from build123d import *

# Parameters (mm, degrees)
IZIM1_R                     = 1.5
IZIM1_R_2                   = 1.5621
IZIM1_R_3                   = 2.5
Y_KSEKLIK_EKSTR_ZYON1_DEPTH = 3


with BuildPart() as part:
    # Çizim1 → Yükseklik-Ekstrüzyon1 (new body)
    with BuildSketch(Plane(origin=(0, 0, 0), x_dir=(1, 0, 0), z_dir=(0, 1, 0))):
        with BuildLine():
            Line((-78.950997289, 12.5), (-73.950997289, 12.5))
            ThreePointArc((-73.950997289, 12.5), (-53.033008589, 53.033008589), (-12.5, 73.950997289))
            Line((-12.5, 73.950997289), (-12.5, 78.950997289))
            ThreePointArc((-12.5, 78.950997289), (0, 91.450997289), (12.5, 78.950997289))
            Line((12.5, 78.950997289), (12.5, 73.950997289))
            ThreePointArc((12.5, 73.950997289), (53.033008589, 53.033008589), (73.950997289, 12.5))
            Line((73.950997289, 12.5), (78.950997289, 12.5))
            ThreePointArc((78.950997289, 12.5), (91.450997289, 0), (78.950997289, -12.5))
            Line((78.950997289, -12.5), (73.950997289, -12.5))
            ThreePointArc((73.950997289, -12.5), (53.033008589, -53.033008589), (12.5, -73.950997289))
            Line((12.5, -73.950997289), (12.5, -78.950997289))
            ThreePointArc((12.5, -78.950997289), (0, -91.450997289), (-12.5, -78.950997289))
            Line((-12.5, -78.950997289), (-12.5, -73.950997289))
            ThreePointArc((-12.5, -73.950997289), (-53.033008589, -53.033008589), (-73.950997289, -12.5))
            Line((-73.950997289, -12.5), (-78.950997289, -12.5))
            ThreePointArc((-78.950997289, -12.5), (-91.450997289, 0), (-78.950997289, 12.5))
        make_face()
        with Locations(Location((-78.950997289, 0, 0), (0, 0, 270))):
            Circle(IZIM1_R, mode=Mode.SUBTRACT)
        with Locations(Location((-78.950997289, 5, 0), (0, 0, 270))):
            Circle(IZIM1_R, mode=Mode.SUBTRACT)
        with Locations(Location((-83.950997289, 0, 0), (0, 0, 270))):
            Circle(IZIM1_R, mode=Mode.SUBTRACT)
        with Locations(Location((-73.950997289, 0, 0), (0, 0, 270))):
            Circle(IZIM1_R, mode=Mode.SUBTRACT)
        with Locations(Location((-78.950997289, -5, 0), (0, 0, 270))):
            Circle(IZIM1_R, mode=Mode.SUBTRACT)
        with Locations(Location((36.071585404, 20.719390461, 0), (0, 0, 270))):
            Circle(IZIM1_R_2, mode=Mode.SUBTRACT)
        with Locations(Location((43.564585404, -27.616809539, 0), (0, 0, 270))):
            Circle(IZIM1_R_2, mode=Mode.SUBTRACT)
        with Locations(Location((-39.061614596, -27.616809539, 0), (0, 0, 270))):
            Circle(IZIM1_R_2, mode=Mode.SUBTRACT)
        with Locations(Location((-39.061614596, 20.719390461, 0), (0, 0, 270))):
            Circle(IZIM1_R_2, mode=Mode.SUBTRACT)
        with Locations(Location((-5, 78.950997289, 0), (0, 0, 270))):
            Circle(IZIM1_R, mode=Mode.SUBTRACT)
        with Locations(Location((0, 78.950997289, 0), (0, 0, 270))):
            Circle(IZIM1_R, mode=Mode.SUBTRACT)
        with Locations(Location((0, 83.950997289, 0), (0, 0, 270))):
            Circle(IZIM1_R, mode=Mode.SUBTRACT)
        with Locations(Location((5, 78.950997289, 0), (0, 0, 270))):
            Circle(IZIM1_R, mode=Mode.SUBTRACT)
        with Locations(Location((0, 73.950997289, 0), (0, 0, 270))):
            Circle(IZIM1_R, mode=Mode.SUBTRACT)
        with Locations(Location((78.950997289, 5, 0), (0, 0, 270))):
            Circle(IZIM1_R, mode=Mode.SUBTRACT)
        with Locations(Location((78.950997289, 0, 0), (0, 0, 270))):
            Circle(IZIM1_R, mode=Mode.SUBTRACT)
        with Locations(Location((83.950997289, 0, 0), (0, 0, 270))):
            Circle(IZIM1_R, mode=Mode.SUBTRACT)
        with Locations(Location((78.950997289, -5, 0), (0, 0, 270))):
            Circle(IZIM1_R, mode=Mode.SUBTRACT)
        with Locations(Location((73.950997289, 0, 0), (0, 0, 270))):
            Circle(IZIM1_R, mode=Mode.SUBTRACT)
        with Locations(Location((5, -78.950997289, 0), (0, 0, 270))):
            Circle(IZIM1_R, mode=Mode.SUBTRACT)
        with Locations(Location((0, -78.950997289, 0), (0, 0, 270))):
            Circle(IZIM1_R, mode=Mode.SUBTRACT)
        with Locations(Location((0, -83.950997289, 0), (0, 0, 270))):
            Circle(IZIM1_R, mode=Mode.SUBTRACT)
        with Locations(Location((-5, -78.950997289, 0), (0, 0, 270))):
            Circle(IZIM1_R, mode=Mode.SUBTRACT)
        with Locations(Location((0, -73.950997289, 0), (0, 0, 270))):
            Circle(IZIM1_R, mode=Mode.SUBTRACT)
        with Locations(Location((45, 45, 0), (0, 0, 270))):
            Circle(IZIM1_R_3, mode=Mode.SUBTRACT)
        with Locations(Location((45, -45, 0), (0, 0, 270))):
            Circle(IZIM1_R_3, mode=Mode.SUBTRACT)
        with Locations(Location((-45, -45, 0), (0, 0, 270))):
            Circle(IZIM1_R_3, mode=Mode.SUBTRACT)
        with Locations(Location((-45, 45, 0), (0, 0, 270))):
            Circle(IZIM1_R_3, mode=Mode.SUBTRACT)
    extrude(amount=Y_KSEKLIK_EKSTR_ZYON1_DEPTH)


solid = part.part
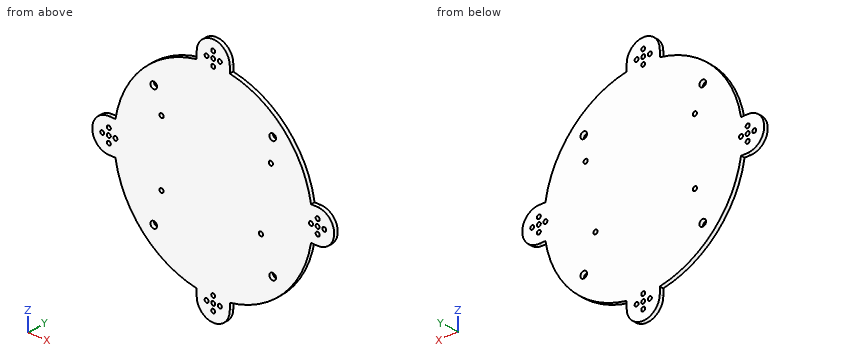
Source: CAD feature listing. Evaluate the final solid. Frame: model axes, mm. Give positions to 0.01 mm unless a question says otherwise; leave off trailing zeros. Write each loop counter-clockwise with the first axis right and the second up, starting at its lowest first coordinate (ties: lowest second). Pieces come first, ordered by that corner, then holes. Notation, with made-up numbers: M 17,-5 L 59,-5 A18 cw 59,6 Z; hole C -23,80 d5. An arc over 180 degrees is marked long. Return JSON: item names as keys, results as strings. Group by question number.
1) Cut plane D-D, the plane y = 0.85. Give the number of separate pieces and of enclosed holes in the cut face, plus the area to 3 significant figures.
2) Cut plane A-A, the plane z = 45. Output: boundary loops of the cut face in (x, y).
3) Cut plane C-C, the plane z = 68.5. Output: boundary loops of the cut face in (x, y), plus the area to 3 significant figures.
4) Material intervals for line 1 along Z through (x, y) = (79, 1.7); line 2 along X through (y, z) = (2, -20) (3 decimals); line 3 along X through (y, z) = (1.45, -45), sorted ascending. Write a range as [from, to].
5) Pin query (flat end, axial travel): P1, Ø0.9, axis at y = 1.5, z = 76, coming from the -X side; P2, Ø1.5, axis at y = 2.5, z = 30, coming from the -X side; P3, Ø1.5, axis at y = 1.5, z = -76.5, coming from the +X side. Return the tip coordinate at first contact, or that it passes through.
6) Cut plane B-B, the plane x = -18. Output: boundary loops of the cut face in (y, z), plus the area to 3 significant figures.
Recorded:
{
 "1": {"separate pieces": "1", "enclosed holes": "28", "area": "18,800 mm²"},
 "2": {"outline": "M -60,0 L -47.5,0 L -47.5,3 L -60,3 Z; M -42.5,0 L 42.5,0 L 42.5,3 L -42.5,3 Z; M 47.5,0 L 60,0 L 60,3 L 47.5,3 Z"},
 "3": {"outline": "M -30.54,0 L 30.54,0 L 30.54,3 L -30.54,3 Z", "area": "183 mm²"},
 "4": {"line 1": "z = [-12.5, -6.5], [-3.5, -1.5], [1.5, 3.5], [6.5, 12.5]", "line 2": "x = [-72.284, -40.448], [-37.675, 34.685], [37.458, 72.284]", "line 3": "x = [-60, -47.5], [-42.5, 42.5], [47.5, 60]"},
 "5": {"P1": "stops at x = -12.5", "P2": "stops at x = -69.06", "P3": "stops at x = 12.5"},
 "6": {"outline": "M 0,-72.81 L 3,-72.81 L 3,72.81 L 0,72.81 Z", "area": "437 mm²"}
}
